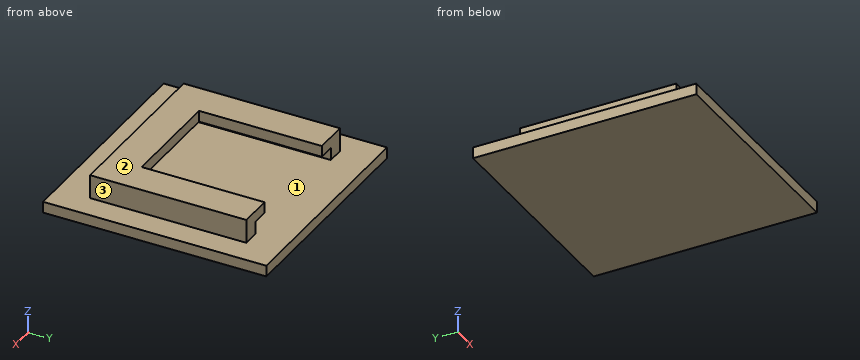
Autodesk Inventor part; units mm, degrees
ref_plane "YZ Plane" through (0, 0, 0) normal (1, 0, 0) x (0, 1, 0)
ref_plane "XZ Plane" through (0, 0, 0) normal (0, 1, 0) x (-1, 0, 0)
ref_plane "XY Plane" through (0, 0, 0) normal (0, 0, 1) x (1, 0, 0)
sketch "Sketch1" plane through (0, 0, 0) normal (0, 0, 1) x (1, 0, 0)
  line L0 (0, 0) -> (80, 0)
  line L1 (80, 0) -> (80, 80)
  line L2 (80, 80) -> (0, 80)
  line L3 (0, 80) -> (0, 0)
  dimension "d0" = 80
  dimension "d1" = 80
extrude "Extrusion1" add sketch "Sketch1" along normal blind 4
sketch "Sketch2" plane through (0, 0, 4) normal (0, 0, 1) x (1, 0, 0)
  line L0 (0, 0) -> (80, 0)
  line L1 (80, 0) -> (80, 80)
  line L2 (9, 68) -> (9, 12)
  line L3 (9, 12) -> (71, 12)
  line L4 (71, 12) -> (71, 68)
  line L5 (71, 68) -> (65, 68)
  line L6 (65, 68) -> (65, 18)
  line L7 (65, 18) -> (15, 18)
  line L8 (15, 18) -> (15, 68)
  line L9 (15, 68) -> (9, 68)
  dimension "d4" = 6
  dimension "d5" = 6
  dimension "d6" = 50
  dimension "d7" = 50
  dimension "d8" = 9
  dimension "d9" = 12
extrude "Extrusion2" add sketch "Sketch2" along normal blind 4.5
sketch "Sketch3" plane through (0, 0, 8.5) normal (0, 0, 1) x (1, 0, 0)
  line L0 (9, 68) -> (9, 12)
  line L1 (9, 12) -> (71, 12)
  line L2 (71, 12) -> (71, 68)
  line L3 (71, 68) -> (65, 68)
  line L4 (65, 68) -> (65, 18)
  line L5 (65, 18) -> (15, 18)
  line L6 (15, 18) -> (15, 68)
  line L7 (15, 68) -> (9, 68)
  line L8 (15, 68) -> (21, 68)
  line L9 (21, 68) -> (21, 24)
  line L10 (21, 24) -> (59, 24)
  line L11 (59, 24) -> (59, 68)
  line L12 (59, 68) -> (65, 68)
  point P0 (0, 0)
  dimension "d12" = 6
  dimension "d13" = 6
extrude "Extrusion3" add sketch "Sketch3" along normal blind 4
properties part number "SpoolHolderSplitBase"
Work out the finished part from the listing and answer in its coordinate system (mm). Face numbers are marked on the shaded views. Give positions to 0.01 mm unless a question says otherwise; leave off trailing zeros. Loops run counter-clockwise (first coordinate to the right, second up) from the corner with the lowest first, then second, coordinate; pieces in that order, holes last. Notation, with made-up numbers: M -20.5,-36 L 37.5,-36 A19 cw 37.5,-5 Z; hole C 45,22 d4. An arc over 180 degrees is marked long. Use CSV: the item, a comma, the result in double quotes.
1) Find section C-C on y = 44.5. Write down the section's boundary in (x, z).
Answer:
outline,"M 0,0 L 80,0 L 80,4 L 71,4 L 71,12.5 L 59,12.5 L 59,8.5 L 65,8.5 L 65,4 L 15,4 L 15,8.5 L 21,8.5 L 21,12.5 L 9,12.5 L 9,4 L 0,4 Z"
2) Find section D-D on y = 75.5. Write down the section's boundary in (x, z).
Answer:
outline,"M 0,0 L 80,0 L 80,4 L 0,4 Z"
3) Find section A-A on z = 10.5. Write down the section's boundary in (x, y), plus the area to 3 significant figures.
Answer:
outline,"M 9,12 L 71,12 L 71,68 L 59,68 L 59,24 L 21,24 L 21,68 L 9,68 Z"
area,"1,800 mm^2"
4) Given P1, Ø5, axis at x = 49, y = 66.5, coming from the +Z side; P2, Ø3, axis at y = 50, z = 11, coming from the -X side; P3, Ø4, axis at y = 42.5, z = 9.5, coming from the +X side, each flat-ended and moving along its own axis, determine where each tip first touches the part or whether it passes through.
Answer:
P1,"z = 4"
P2,"x = 9"
P3,"x = 71"
5) Find section B-B on x = 17. Write down the section's boundary in (y, z).
Answer:
outline,"M 0,0 L 80,0 L 80,4 L 18,4 L 18,8.5 L 68,8.5 L 68,12.5 L 12,12.5 L 12,4 L 0,4 Z"
6) Determine the mould class of the marked faces 1, 2 and 3 for opening direction X: released by +X, released by -X, zero draft, split by the parting line, or undercut.
Answer:
face 1,"undercut"
face 2,"zero draft"
face 3,"released by +X"
7) Consider L1, parallel to X at y = 37.5, z = 10; L2, parallel to Z at x = 16.5, y = 64; L3, parallel to X at y = 53.5, z = 7. Determine where each line is inside the solid, lowest interval first.
Answer:
L1,"9 to 21, 59 to 71"
L2,"0 to 4, 8.5 to 12.5"
L3,"9 to 15, 65 to 71"
